CAD build for the part. Positions are in the model's coordinates, mm. Face numbers are marked on the shaded views. A direction names the side the tool comes from. Coordinates: 2 decimals unless noted, no trailing zeros. Write each loop counter-clockwise with the first axis right and the second up, starting at its lowest first coordinate (ties: lowest second). Pieces come first, ordered by that corner, then holes.
```python
from build123d import *

# Parameters (mm, degrees)
F0_W     = 101.6
F0_H     = 101.6
F1_DEPTH = 19.05
F3_DEPTH = 101.601
F5_DEPTH = 101.601
F6_W     = 101.6
F6_H     = 3.175
F7_DEPTH = 101.601


with BuildPart() as f1:
    # F0 (on Top) → F1 (new body)
    with BuildSketch(Plane.XY):
        Rectangle(F0_W, F0_H)
    extrude(amount=F1_DEPTH)

    # F2 (on face) → F3 (cut, through all)
    with BuildSketch(Plane.YZ.offset(50.8)):
        Polygon((6.223, 19.05), (-6.223, 19.05), (-12.7635, 2.54), (12.7635, 2.54), align=None)
    extrude(amount=-F3_DEPTH, mode=Mode.SUBTRACT)

    # F4 (on face) → F5 (cut, through all)
    with BuildSketch(Plane.XZ.offset(50.8)):
        Polygon((6.223, 19.05), (-6.223, 19.05), (-12.7635, 2.54), (12.7635, 2.54), align=None)
    extrude(amount=-F5_DEPTH, mode=Mode.SUBTRACT)

    # F6 (on face) → F7 (cut, through all)
    with BuildSketch(Plane.YZ.offset(50.8)):
        with Locations((0, 17.4625)):
            Rectangle(F6_W, F6_H)
    extrude(amount=-F7_DEPTH, mode=Mode.SUBTRACT)


solid = f1.part
```
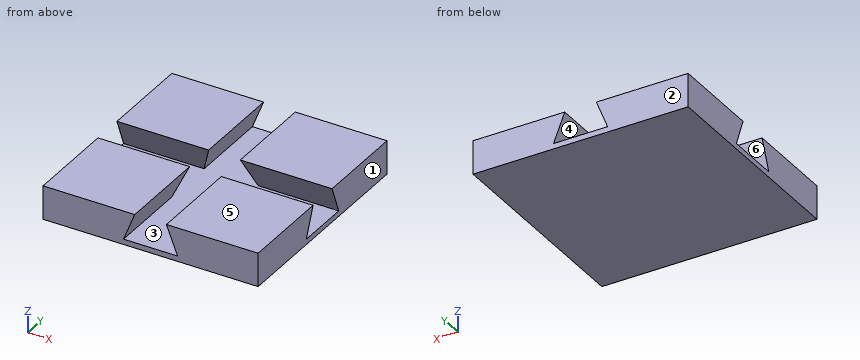
Item 1: Which spindle directions (+Z, -Z, +X, -X, +Y, -Y) get a long thin tool onto all of the face, cutting with end or side? Do the marked faces 4, 5 and 6. Say none if no direction does.
Item 2: Two-plate mould, pull along X, no slides. Class the marked faces 1, 2 and 3: +X half, -X half, draft (parallel to the pull), parting line (faces both ways), or undercut.
Item 3: Saw through at C-C, the plane z = 11.25. Write the cut outline in (x, y).
Item 4: Saw through at B-B, the plane y = -11. Write the cut outline in (x, z) (3 decimals).
Item 5: Wall check: line 1 along X through (y, z) = (-34.5, 7); line 2 along X through (y, z) = (20, 12); line 3 along Z through (x, y) = (13, 4.5). Give the ranges that are in metal, low to high.
Item 6: Flat gauge pin, fed straight in: pin 1 Ø4 at (x, z) = (9, 5.5) entering from +Y. Where does the tip first touch, or does it go through?
Item 7: Saw through at A-A, the plane x = -28.5. Write the cut outline in (y, z) (1 decimal), and give its area (3 significant figures).
Working result:
1. face 4: +Y, -Y
1. face 5: +Z, +X, -X, +Y, -Y
1. face 6: +X, -X
2. face 1: +X half
2. face 2: draft
2. face 3: undercut
3. outline: (-50.8, -50.8) - (-9.31, -50.8) - (-9.31, -9.31) - (-50.8, -9.31) - close; (-50.8, 9.31) - (-9.31, 9.31) - (-9.31, 50.8) - (-50.8, 50.8) - close; (9.31, -50.8) - (50.8, -50.8) - (50.8, -9.31) - (9.31, -9.31) - close; (9.31, 9.31) - (50.8, 9.31) - (50.8, 50.8) - (9.31, 50.8) - close
4. outline: (-50.8, 0) - (50.8, 0) - (50.8, 2.54) - (-50.8, 2.54) - close; (-50.8, 6.992) - (-11, 6.992) - (-7.481, 15.875) - (-50.8, 15.875) - close; (7.481, 15.875) - (11, 6.992) - (50.8, 6.992) - (50.8, 15.875) - close
5. line 1: x = -50.8 to -11, 11 to 50.8
5. line 2: x = -50.8 to -9.02, 9.02 to 50.8
5. line 3: z = 0 to 2.54
6. pin 1: passes through
7. outline: (-50.8, 0) - (50.8, 0) - (50.8, 15.9) - (7.5, 15.9) - (12.8, 2.5) - (-12.8, 2.5) - (-7.5, 15.9) - (-50.8, 15.9) - close
7. area: 1,340 mm2
